The model under review builds one solid part; all positions refer to its coordinate system, in mm. Face numbers are marked on the shaded views. Round coordinates to 2 decimals unless told otherwise and drop trailing zeros. Loops run counter-clockwise (first coordinate to the right, second up) from the corner with the lowest first, then second, coordinate; pieces in that order, holes last. Notation, with made-up numbers: (-25.75, 82) - (-11.75, 82) arc R14 cw to (-11.75, 98) - close; hole circle Ø5 at (1.5, -6.5). An arc over 180 degrees is marked (long way). Answer as CSV lines item,"result".
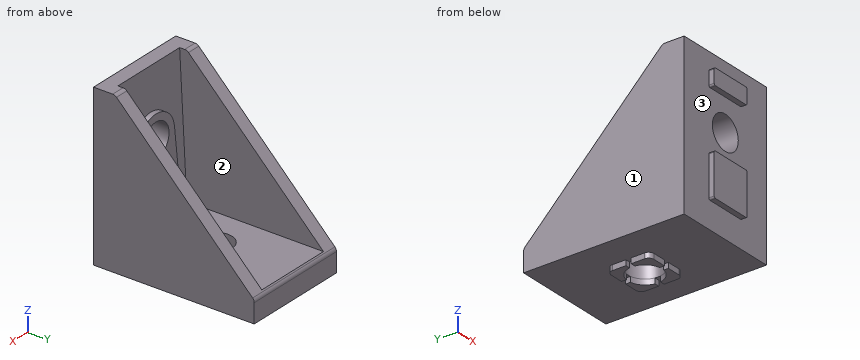
from build123d import *
from build123d.topology import SkipClean

# Parameters (mm, degrees)
BOSS_EXTRUDE1_DEPTH      = 10
BOSS_EXTRUDE1_DEPTH_BACK = 10
CUT_EXTRUDE1_DEPTH       = 7.5
CUT_EXTRUDE1_DEPTH_BACK  = 7.5
BOSS_EXTRUDE2_DEPTH      = 2
SKETCH4_R                = 3.15
CUT_EXTRUDE2_DEPTH       = 5
SKETCH5_R                = 3.15
CUT_EXTRUDE3_DEPTH       = 4
SKETCH6_W                = 20
SKETCH6_H                = 30
BOSS_EXTRUDE3_DEPTH      = 1
SKETCH7_W                = 20
SKETCH7_H                = 30
CUT_EXTRUDE4_DEPTH       = 1
SKETCH8_W                = 20
SKETCH8_H                = 30
BOSS_EXTRUDE4_DEPTH      = 1
CUT_EXTRUDE5_START       = -1
SKETCH9_W                = 20
SKETCH9_H                = 30
CUT_EXTRUDE5_DEPTH       = 1


with BuildPart() as part:
    # Sketch1 → Boss-Extrude1 (new, two sides: drawn at the far end of the back side and taken through both)
    with BuildSketch(Plane(origin=(0, 0, 0), x_dir=(0, 0, -1), z_dir=(1, 0, 0)).offset(-BOSS_EXTRUDE1_DEPTH_BACK)):
        with BuildLine():
            Line((-30, 0), (0, 0))
            Line((0, 0), (0, 30))
            Line((0, 30), (-3.585786438, 30))
            ThreePointArc((-3.585786438, 30), (-3.96846987, 29.923879533), (-4.292893219, 29.707106781))
            Line((-4.292893219, 29.707106781), (-29.707106781, 4.292893219))
            ThreePointArc((-29.707106781, 4.292893219), (-29.923879533, 3.96846987), (-30, 3.585786438))
            Line((-30, 3.585786438), (-30, 0))
        make_face()
    extrude(amount=BOSS_EXTRUDE1_DEPTH + BOSS_EXTRUDE1_DEPTH_BACK)

    # Sketch2 → Cut-Extrude1 (cut, two sides: drawn at the far end of the back side and taken through both)
    with BuildSketch(Plane(origin=(0, 0, 0), x_dir=(0, 0, -1), z_dir=(1, 0, 0)).offset(-CUT_EXTRUDE1_DEPTH_BACK)):
        Polygon((-34, 2.427766622), (-4.5, 3.97379611), (-4.5, 34), (-34, 34), align=None)
    extrude(amount=CUT_EXTRUDE1_DEPTH + CUT_EXTRUDE1_DEPTH_BACK, mode=Mode.SUBTRACT)

    # Sketch3 → Boss-Extrude2 (add)
    with BuildSketch(Plane(origin=(0, 4, 0), x_dir=(1, 0, 0), z_dir=(0, 1, 0))):
        with BuildLine():
            Line((-5.420884207, -10.5), (-4.4686916, -18.529901296))
            ThreePointArc((-4.4686916, -18.529901296), (0, -22.5), (4.4686916, -18.529901296))
            Line((4.4686916, -18.529901296), (5.420884207, -10.5))
            Line((5.420884207, -10.5), (-5.420884207, -10.5))
        make_face()
    extrude(amount=-BOSS_EXTRUDE2_DEPTH)

    # Sketch4 → Cut-Extrude2 (cut)
    with BuildSketch(Plane.XY):
        with Locations((0, 15)):
            Circle(SKETCH4_R)
    extrude(amount=CUT_EXTRUDE2_DEPTH, mode=Mode.SUBTRACT)

    # Sketch5 → Cut-Extrude3 (cut)
    with BuildSketch(Plane(origin=(0, 0, 0), x_dir=(1, 0, 0), z_dir=(0, 1, 0))):
        with Locations(Location((0, -18, 0), (0, 0, 270))):
            Circle(SKETCH5_R)
    extrude(amount=CUT_EXTRUDE3_DEPTH, mode=Mode.SUBTRACT)

    # Sketch6 → Boss-Extrude3 (add)
    with BuildSketch(Plane(origin=(0, 0, 0), x_dir=(1, 0, 0), z_dir=(0, 1, 0))):
        with Locations((0, -15)):
            Rectangle(SKETCH6_W, SKETCH6_H)
    extrude(amount=-BOSS_EXTRUDE3_DEPTH)

    # Sketch7 → Cut-Extrude4 (cut)
    with BuildSketch(Plane(origin=(0, 0, 0), x_dir=(1, 0, 0), z_dir=(0, 1, 0))):
        with Locations((0, -15)):
            Rectangle(SKETCH7_W, SKETCH7_H)
        with BuildLine():
            Line((-3.7, -13), (3.7, -13))
            ThreePointArc((3.7, -13), (3.912132034, -12.912132034), (4, -12.7))
            Line((4, -12.7), (4, -5.3))
            ThreePointArc((4, -5.3), (3.912132034, -5.087867966), (3.7, -5))
            Line((3.7, -5), (-3.7, -5))
            ThreePointArc((-3.7, -5), (-3.912132034, -5.087867966), (-4, -5.3))
            Line((-4, -5.3), (-4, -12.7))
            ThreePointArc((-4, -12.7), (-3.912132034, -12.912132034), (-3.7, -13))
        make_face(mode=Mode.SUBTRACT)
        with BuildLine():
            Line((-3.7, -27), (3.7, -27))
            ThreePointArc((3.7, -27), (3.912132034, -26.912132034), (4, -26.7))
            Line((4, -26.7), (4, -24.3))
            ThreePointArc((4, -24.3), (3.912132034, -24.087867966), (3.7, -24))
            Line((3.7, -24), (-3.7, -24))
            ThreePointArc((-3.7, -24), (-3.912132034, -24.087867966), (-4, -24.3))
            Line((-4, -24.3), (-4, -26.7))
            ThreePointArc((-4, -26.7), (-3.912132034, -26.912132034), (-3.7, -27))
        make_face(mode=Mode.SUBTRACT)
    extrude(amount=-CUT_EXTRUDE4_DEPTH, mode=Mode.SUBTRACT)

    # Sketch8 → Boss-Extrude4 (add)
    with BuildSketch(Plane.XY):
        with Locations((0, 15)):
            Rectangle(SKETCH8_W, SKETCH8_H)
    extrude(amount=-BOSS_EXTRUDE4_DEPTH)

    # Sketch9 → Cut-Extrude5 (cut)
    with SkipClean():  # the faces are left unmerged after this step: merging them gives an invalid solid
        with BuildSketch(Plane.XY.offset(CUT_EXTRUDE5_START)):
            with Locations((0, 15)):
                Rectangle(SKETCH9_W, SKETCH9_H)
            with BuildLine():
                Line((0.5, 11), (3, 11))
                ThreePointArc((3, 11), (3.707106781, 11.292893219), (4, 12))
                Line((4, 12), (4, 14.5))
                Line((4, 14.5), (3.110064308, 14.5))
                ThreePointArc((3.110064308, 14.5), (2.227386361, 12.772613639), (0.5, 11.889935692))
                Line((0.5, 11.889935692), (0.5, 11))
            make_face(mode=Mode.SUBTRACT)
            with BuildLine():
                Line((0.5, 19), (0.5, 18.110064308))
                ThreePointArc((0.5, 18.110064308), (2.227386361, 17.227386361), (3.110064308, 15.5))
                Line((3.110064308, 15.5), (4, 15.5))
                Line((4, 15.5), (4, 18))
                ThreePointArc((4, 18), (3.707106781, 18.707106781), (3, 19))
                Line((3, 19), (0.5, 19))
            make_face(mode=Mode.SUBTRACT)
            with BuildLine():
                Line((-3, 11), (-0.5, 11))
                Line((-0.5, 11), (-0.5, 11.889935692))
                ThreePointArc((-0.5, 11.889935692), (-2.227386361, 12.772613639), (-3.110064308, 14.5))
                Line((-3.110064308, 14.5), (-4, 14.5))
                Line((-4, 14.5), (-4, 12))
                ThreePointArc((-4, 12), (-3.707106781, 11.292893219), (-3, 11))
            make_face(mode=Mode.SUBTRACT)
            with BuildLine():
                Line((-4, 15.5), (-3.110064308, 15.5))
                ThreePointArc((-3.110064308, 15.5), (-2.227386361, 17.227386361), (-0.5, 18.110064308))
                Line((-0.5, 18.110064308), (-0.5, 19))
                Line((-0.5, 19), (-3, 19))
                ThreePointArc((-3, 19), (-3.707106781, 18.707106781), (-4, 18))
                Line((-4, 18), (-4, 15.5))
            make_face(mode=Mode.SUBTRACT)
        extrude(amount=CUT_EXTRUDE5_DEPTH, mode=Mode.SUBTRACT)


solid = part.part
1. Take a section at B-B (y = 27.5). State the section outline as (x, z) points, plus the area to 3 significant figures.
Numbers:
outline,"(-10, 0) - (10, 0) - (10, 6.5) - (7.5, 6.5) - (7.5, 4.5) - (-7.5, 4.5) - (-7.5, 6.5) - (-10, 6.5) - close"
area,"100 mm²"
2. Clearance check with flat-ended pins moving along their axes: pin 1 (2 mm diameter, centred on x = 0.5, z = 7.5, fed in from +Y); pin 2 (0.5 mm diameter, centred on x = 0.5, y = -0.5, fed in from -Z); pin 3 (0.5 mm diameter, centred on y = 13.5, z = -0.5, fed in from -X); pin 4 (1.1 mm diameter, centred on y = 13, z = -0.5, fed in from +X). State where each tip first meets the part, or that it passes through.
Numbers:
pin 1,"stops at y = 3.87"
pin 2,"stops at z = 5"
pin 3,"stops at x = -4"
pin 4,"stops at x = 10"
3. Wall thickness on probe 1 along X at (y, z) = (15, 1); probe 2 along Y at (x, z) = (0, 3); probe 3 along X at (y, z) = (5, 14): over which ranges is each line inside the solid? List them lowest first.
Numbers:
probe 1,"x = -10 to -3.15, 3.15 to 10"
probe 2,"y = 0 to 11.85, 18.15 to 30"
probe 3,"x = -10 to -7.5, 7.5 to 10"
4. Take a section at D-D (x = 7). State the section outline as (y, z) points, plus the area to 3 significant figures.
Numbers:
outline,"(0, 0) - (30, 0) - (30, 3.59) arc R1 ccw to (29.71, 4.29) - (29.5, 4.5) - (3.97, 4.5) - (2.64, 30) - (0, 30) - close"
area,"219 mm²"
5. Take a section at C-C (z = 20). State the section outline as (x, y) points.
Numbers:
outline,"(-10, 0) - (-2.43, 0) - (-2.43, 4) - (-4.03, 4) - (-4.03, 3.16) - (-7.5, 3.16) - (-7.5, 14) - (-10, 14) - close; (2.43, 0) - (10, 0) - (10, 14) - (7.5, 14) - (7.5, 3.16) - (4.03, 3.16) - (4.03, 4) - (2.43, 4) - close"
6. Take a section at A-A (x = 0). State the section outline as (y, z) points.
Numbers:
outline,"(-1, 5) - (0, 5) - (0, 0) - (11.85, 0) - (11.85, 4.5) - (3.97, 4.5) - (3.66, 10.5) - (4, 10.5) - (4, 14.85) - (0, 14.85) - (0, 13) - (-1, 13) - close; (-1, 24) - (0, 24) - (0, 21.15) - (4, 21.15) - (4, 22.5) - (3.03, 22.5) - (2.64, 30) - (0, 30) - (0, 27) - (-1, 27) - close; (18.15, 0) - (30, 0) - (30, 3.59) arc R1 ccw to (29.71, 4.29) - (29.5, 4.5) - (18.15, 4.5) - close"
7. Draft analysis for pull direction X (two halves, no side actions). For the marked faces 1, 2 and 3, state which applies: +X half, -X half, draft (parallel to the pull), parting line (faces both ways), or undercut.
Numbers:
face 1,"-X half"
face 2,"undercut"
face 3,"draft"
